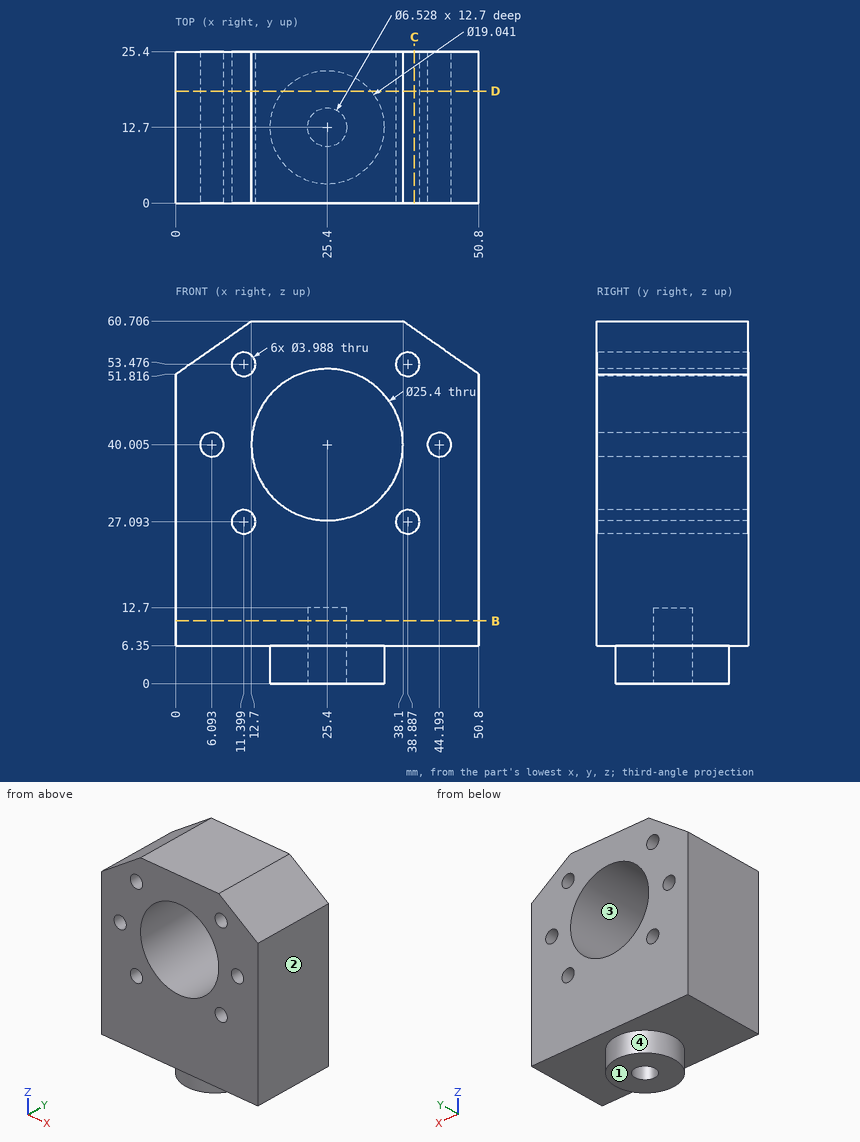
The drawing under review shows one solid part. Ordinate dimensions are in mm from its lowest x, y, z. Give positions to 0.01 mm unless a question says otherwise; leave off trailing zeros. Write each loop counter-clockwise with the first axis right and the second up, starting at its lowest first coordinate (ties: lowest second). Pieces come first, ordered by that corner, then holes. Notation, with made-up numbers: (-28, 24.25) -> (26, 24.25) arc R15 cw to (26, 36.25) -> close; hole circle Ø6 at (66, 80). An arc over 180 degrees is marked (long way). Put each result on its own line as item: value.
(1) For pin 1 Ø2 at (x, y) = (25.5, 13) entering from -Z; pin 2 Ø20.5 at (x, z) = (25.4, 40.005) entering from +Y; pin 3 Ø4 at (y, z) = (9, 28) entering from -X, all flat-tipped, find the tip position at first contact; note any pin that passes through.
Results are:
pin 1: z = 12.7
pin 2: through
pin 3: x = 0
(2) We need section B-B, the plane z = 10.5. Give the boundary of the cut face in (x, y).
Results are:
outline: (0, 0) -> (50.8, 0) -> (50.8, 25.4) -> (0, 25.4) -> close; hole circle Ø6.53 at (25.4, 12.7)
(3) We need section D-D, the plane y = 18.75. State how many separate pieces and enclosed holes the cut face has, and give its area (3 significant figures).
Results are:
separate pieces: 1
enclosed holes: 7
area: 2,160 mm²
(4) We need section C-C, the plane x = 40. Give the boundary of the cut face in (y, z).
Results are:
outline: (0, 6.35) -> (25.4, 6.35) -> (25.4, 25.44) -> (0, 25.44) -> close; (0, 28.75) -> (25.4, 28.75) -> (25.4, 51.82) -> (0, 51.82) -> close; (0, 55.13) -> (25.4, 55.13) -> (25.4, 59.38) -> (0, 59.38) -> close
(5) To check wall thickness, follow probe 1 along X at (y, z) = (14.25, 53.5) (1 decimal); probe 2 along Z at (x, y) = (25.4, 6.25) (1 decimal); probe 3 along X at (y, z) = (13.5, 47). State the ranges of each line that lie inside material, in increasing order. Write a range as from..to.
Results are:
probe 1: 2.4..9.4, 13.4..36.9, 40.9..48.4
probe 2: 0..27.3, 52.7..60.7
probe 3: 0..14.8, 36..50.8
(6) The part is to be moulded in two halves that separate along X. For the marked faces 1, 2, 3 and 4, say which applies: pulls with the +X half, pulls with the -X half, needs draft (parallel to the pull), parting line crosses it, or undercut.
Results are:
face 1: needs draft
face 2: pulls with the +X half
face 3: undercut
face 4: parting line crosses it
